Model file for the job. Use its own axes, mm. Give positions to 0.01 mm unless a question says otherwise; leave off trailing zeros. Loops run counter-clockwise (first coordinate to the right, second up) from the corner with the lowest first, then second, coordinate; pieces in that order, holes last. Notation, with made-up numbers: (2.5, -19) - (25.5, -19) arc R19 cw to (25.5, 13) - close; hole circle Ø2 at (-34, 68.25). An arc over 180 degrees is marked (long way). Answer as CSV lines item,"result". Start each with the question number.
Item 1: Saw through at C-C on x = 28.54. Give the cut face in (y, z), plus the area to 3 significant figures.
Item 2: Saw through at D-D on z = 0. Give the cut face in (x, y), plus the area to 3 significant figures.
Item 3: Drill centre lines: L1, parallel to X at y = 0.55, z = 0; L2, parallel to X at y = 0.35, z = 14; L3, parallel to X at y = 1.55, z = 28. Where is each one in solid material? Low to high. Write a range as from..to.
Item 4: Saw through at A-A on z = 14. Give the cut face in (x, y), plus the area to 3 significant figures.
Item 5: Pull direction Z, two halves, no side cores. Call faces 1 (the cylindrical face through (41.897, 0.986, 29.21)), 2 (the cylindrical face through (26.912, 1.72, 17.926)), 3 (the cylindrical face through (20.35, 1.699, 33.715)), 4 (the flat face through (19.7, 0.5, -6)): pulls with the +Z half, pulls with the -Z half, needs draft (parallel to the pull), parting line crosses it, or undercut.
Item 6: Saw through at B-B on x = 40. Give the cut face in (y, z).
from build123d import *

# Parameters (mm, degrees)
SKETCH2_W           = 50
SKETCH2_H           = 40
SKETCH2_R           = 2.25
BOSS_EXTRUDE1_DEPTH = 2
CUT_EXTRUDE3_REACH  = 58.436
SKETCH4_R           = 4.25
FILLET2_R           = 1


with BuildPart() as part:
    # Sketch2 → Boss-Extrude1 (new body)
    with BuildSketch(Plane(origin=(0, 0, 0), x_dir=(1, 0, 0), z_dir=(0, 1, 0))):
        with Locations((20, -14)):
            Rectangle(SKETCH2_W, SKETCH2_H)
        with Locations(Location((0, 0, 0), (0, 0, 270))):
            Circle(SKETCH2_R, mode=Mode.SUBTRACT)
        with Locations(Location((40, 0, 0), (0, 0, 270))):
            Circle(SKETCH2_R, mode=Mode.SUBTRACT)
        with Locations(Location((0, -28, 0), (0, 0, 270))):
            Circle(SKETCH2_R, mode=Mode.SUBTRACT)
        with Locations(Location((40, -28, 0), (0, 0, 270))):
            Circle(SKETCH2_R, mode=Mode.SUBTRACT)
    extrude(amount=BOSS_EXTRUDE1_DEPTH)

    # Sketch4 → Cut-Extrude3 (cut, up to next)
    with BuildSketch(Plane(origin=(0, 2, 0), x_dir=(1, 0, 0), z_dir=(0, 1, 0)), mode=Mode.PRIVATE) as cut_extrude3_sk1:
        with Locations(Location((28.54, -14, 0), (0, 0, 270))):
            Circle(SKETCH4_R)
    cut_extrude3_tool1 = extrude(cut_extrude3_sk1.sketch, amount=-CUT_EXTRUDE3_REACH, mode=Mode.PRIVATE) & part.part
    add(cut_extrude3_tool1.solids().sort_by_distance((28.54, 2, 14))[0], mode=Mode.SUBTRACT)

    # Sketch7 → Cut-Revolve1 (revolve, cut)
    with BuildSketch(Plane(origin=(0, 0, 14), x_dir=(-1, 0, 0), z_dir=(0, 0, -1)), mode=Mode.PRIVATE) as cut_revolve1_sk:
        with BuildLine():
            Line((-24.54, 1.5), (-24.54, 0.5))
            ThreePointArc((-24.54, 0.5), (-24.04, 1), (-24.54, 1.5))
        make_face()
    revolve(cut_revolve1_sk.sketch.rotate(Axis((28.54, 2, 14), (0, -1, 0)), 270), axis=Axis((28.54, 2, 14), (0, -1, 0)), mode=Mode.SUBTRACT)

    # Fillet2
    fillet2_edges = [part.edges().sort_by_distance(p)[0] for p in [
        (45, 2, 14),
        (20, 2, -6),
        (-5, 2, 14),
        (20, 2, 34),
    ]]
    fillet(fillet2_edges, radius=FILLET2_R)


solid = part.part
Responses:
1,outline,"(0, -6) - (1, -6) arc R1 ccw to (2, -5) - (2, 9.75) - (1.43, 9.75) arc R0.5 cw to (0.57, 9.75) - (0, 9.75) - close; (0, 18.25) - (0.57, 18.25) arc R0.5 cw to (1.43, 18.25) - (2, 18.25) - (2, 33) arc R1 ccw to (1, 34) - (0, 34) - close"
1,area,"62.3 mm2"
2,outline,"(-5, 0) - (-2.25, 0) - (-2.25, 2) - (-4, 2) arc R1 ccw to (-5, 1) - close; (2.25, 0) - (37.75, 0) - (37.75, 2) - (2.25, 2) - close; (42.25, 0) - (45, 0) - (45, 1) arc R1 ccw to (44, 2) - (42.25, 2) - close"
2,area,"81.6 mm2"
3,L1,"-5..-2.25, 2.25..37.75, 42.25..45"
3,L2,"-5..24.29, 32.79..45"
3,L3,"-4.84..-2.25, 2.25..37.75, 42.25..44.84"
4,outline,"(-5, 0) - (24.29, 0) - (24.29, 0.57) arc R0.5 cw to (24.29, 1.43) - (24.29, 2) - (-4, 2) arc R1 ccw to (-5, 1) - close; (32.79, 0) - (45, 0) - (45, 1) arc R1 ccw to (44, 2) - (32.79, 2) - (32.79, 1.43) arc R0.5 cw to (32.79, 0.57) - close"
4,area,"82.3 mm2"
5,face 1,"undercut"
5,face 2,"undercut"
5,face 3,"pulls with the +Z half"
5,face 4,"pulls with the -Z half"
6,outline,"(0, -6) - (1, -6) arc R1 ccw to (2, -5) - (2, -2.25) - (0, -2.25) - close; (0, 2.25) - (2, 2.25) - (2, 25.75) - (0, 25.75) - close; (0, 30.25) - (2, 30.25) - (2, 33) arc R1 ccw to (1, 34) - (0, 34) - close"
